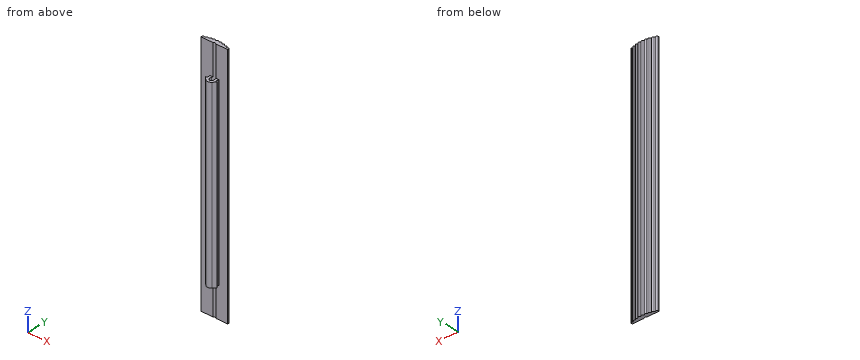
from build123d import *

# Parameters (mm, degrees)
BOSS_EXTRUDE2_DEPTH = 203.2
CUT_EXTRUDE1_REACH  = 357.917
SKETCH2_W           = 22.225
SKETCH2_H           = 25.4


with BuildPart() as part:
    # Sketch1 → Boss-Extrude2 (new body)
    with BuildSketch(Plane.XY.offset(152.4)):
        with BuildLine():
            Line((-11.1125, 7.155754294), (-11.1125, 6.2992))
            Line((-11.1125, 6.2992), (-4.0132, 6.2992))
            ThreePointArc((-4.0132, 6.2992), (-3.653989755, 6.150410245), (-3.5052, 5.7912))
            Line((-3.5052, 5.7912), (-3.5052, 3.980754294))
            ThreePointArc((-3.5052, 3.980754294), (-3.653989755, 3.621544049), (-4.0132, 3.472754294))
            Line((-4.0132, 3.472754294), (-4.7625, 3.472754294))
            Line((-4.7625, 3.472754294), (-2.563540889, 1.114659348))
            ThreePointArc((-2.563540889, 1.114659348), (1.91e-07, 0), (2.563541217, 1.114659472))
            Line((2.563541217, 1.114659472), (4.7625, 3.472754294))
            Line((4.7625, 3.472754294), (4.0132, 3.472754294))
            ThreePointArc((4.0132, 3.472754294), (3.653989755, 3.621544049), (3.5052, 3.980754294))
            Line((3.5052, 3.980754294), (3.5052, 5.7912))
            ThreePointArc((3.5052, 5.7912), (3.653989755, 6.150410245), (4.0132, 6.2992))
            Line((4.0132, 6.2992), (11.1125, 6.2992))
            Line((11.1125, 6.2992), (11.1125, 7.155754292))
            ThreePointArc((11.1125, 7.155754292), (10.663537153, 7.928210313), (9.770119113, 7.920454737))
            ThreePointArc((9.770119113, 7.920454737), (9.148763616, 7.659085907), (8.642363834, 8.104007899))
            ThreePointArc((8.642363834, 8.104007899), (8.019118897, 8.901877), (7.05308944, 8.59886472))
            ThreePointArc((7.05308944, 8.59886472), (6.504535766, 8.494192995), (6.085440415, 8.863281588))
            ThreePointArc((6.085440415, 8.863281588), (5.452899276, 9.555232733), (4.552056662, 9.295642159))
            ThreePointArc((4.552056662, 9.295642159), (3.931317659, 9.028192281), (3.421209266, 9.471628606))
            ThreePointArc((3.421209266, 9.471628606), (2.68084511, 9.976690828), (1.876956272, 9.580471612))
            ThreePointArc((1.876956272, 9.580471612), (1.327001325, 9.29621405), (0.796430567, 9.615192851))
            ThreePointArc((0.796430567, 9.615192851), (-2e-09, 10.1092), (-0.796430568, 9.615192848))
            ThreePointArc((-0.796430568, 9.615192848), (-1.327001326, 9.29621405), (-1.876956272, 9.580471612))
            ThreePointArc((-1.876956272, 9.580471612), (-2.680845114, 9.976690828), (-3.421209269, 9.471628598))
            ThreePointArc((-3.421209269, 9.471628598), (-3.931317662, 9.028192282), (-4.552056659, 9.295642158))
            ThreePointArc((-4.552056659, 9.295642158), (-5.45289928, 9.555232733), (-6.085440418, 8.863281574))
            ThreePointArc((-6.085440418, 8.863281574), (-6.504535766, 8.494192992), (-7.053089431, 8.59886471))
            ThreePointArc((-7.053089431, 8.59886471), (-8.019118881, 8.901877006), (-8.642363831, 8.104007918))
            ThreePointArc((-8.642363831, 8.104007918), (-9.148763609, 7.659085911), (-9.770119113, 7.920454739))
            ThreePointArc((-9.770119113, 7.920454739), (-10.663537153, 7.928210315), (-11.1125, 7.155754294))
        make_face()
        with BuildLine():
            Line((-1.5875, 3.472754294), (-1.5875, 5.276154294))
            ThreePointArc((-1.5875, 5.276154294), (0, 6.863654294), (1.5875, 5.276154294))
            Line((1.5875, 5.276154294), (1.5875, 3.472754294))
            ThreePointArc((1.5875, 3.472754294), (0, 1.885254294), (-1.5875, 3.472754294))
        make_face(mode=Mode.SUBTRACT)
    extrude(amount=BOSS_EXTRUDE2_DEPTH)

    # Cut-Extrude1: up to this face of the body (flat: up to its plane)
    cut_extrude1_end = Plane(part.part.faces().sort_by_distance((7.56285, 6.2992, 254))[0])
    # Sketch2 → Cut-Extrude1 (cut, up to the picked face)
    with BuildSketch(Plane(origin=(0, 0, 0), x_dir=(1, 0, 0), z_dir=(0, 1, 0)), mode=Mode.PRIVATE) as cut_extrude1_sk1:
        with Locations((0, -165.1)):
            Rectangle(SKETCH2_W, SKETCH2_H)
    cut_extrude1_tool1 = split(extrude(cut_extrude1_sk1.sketch, amount=CUT_EXTRUDE1_REACH, mode=Mode.PRIVATE), bisect_by=cut_extrude1_end, keep=Keep.BOTH, mode=Mode.PRIVATE)
    # Sketch2 → Cut-Extrude1 (cut, up to the picked face)
    with BuildSketch(Plane(origin=(0, 0, 0), x_dir=(1, 0, 0), z_dir=(0, 1, 0)), mode=Mode.PRIVATE) as cut_extrude1_sk2:
        with Locations((0, -342.9)):
            Rectangle(SKETCH2_W, SKETCH2_H)
    cut_extrude1_tool2 = split(extrude(cut_extrude1_sk2.sketch, amount=CUT_EXTRUDE1_REACH, mode=Mode.PRIVATE), bisect_by=cut_extrude1_end, keep=Keep.BOTH, mode=Mode.PRIVATE)
    add(cut_extrude1_tool1.solids().sort_by(Axis((0, 0, 165.1), (0, 1, 0)))[0], mode=Mode.SUBTRACT)
    add(cut_extrude1_tool2.solids().sort_by(Axis((0, 0, 342.9), (0, 1, 0)))[0], mode=Mode.SUBTRACT)


solid = part.part
Check sheet for the modelled part. Datum: model origin and axes. Units: mm. Give positions to 0.01 mm unless a question says otherwise; leave off trailing zeros. Write each loop counter-clockwise with the first axis right and the second up, starting at its lowest first coordinate (ties: lowest second). Pieces come first, ordered by that corner, then holes. Notation, with made-up numbers: M 33.5,20 L 92.5,20 A24 cw 92.5,44 Z; hole C -21,67.25 d7. An arc over 180 degrees is marked long. Use one line per item in the form item = value.
(1) Depth check by flat-ended pin: P1, Ø3, axis at x = -7, z = 221, coming from the +Y side; P2, Ø11, axis at x = 6, z = 292, coming from the -Y side; P3, Ø0.5, axis at y = 5, z = 227, coming from the -X side. Enter the tip coordinate at first touch or a pass-through.
Answer block:
P1 = 9.54
P2 = 0.04
P3 = -3.51
(2) Material ranges on line 1 along X through (y, z) = (5.5, 216); line 2 along X through (y, z) = (7.75, 330); line 3 along X through (y, z) = (8.75, 205.5), recorded low to high.
Answer block:
line_1 = -3.51 to -1.57, 1.57 to 3.51
line_2 = -10.88 to -9.59, -8.91 to 8.91, 9.59 to 10.88
line_3 = -8.31 to -7.2, -6.15 to 6.15, 7.2 to 8.31
(3) Section check A-A on z = 333. Record the boundary of the cut face in (x, y) (1 decimal), plus the area to 3 significant figures.
Answer block:
outline = M -11.1,6.3 L -1.2,6.3 A1.6 cw 1.2,6.3 L 11.1,6.3 L 11.1,7.2 A0.9 ccw 9.8,7.9 A0.6 cw 8.6,8.1 A0.9 ccw 7.1,8.6 A0.6 cw 6.1,8.9 A0.9 ccw 4.6,9.3 A0.6 cw 3.4,9.5 A0.9 ccw 1.9,9.6 A0.6 cw 0.8,9.6 A0.9 ccw -0.8,9.6 A0.6 cw -1.9,9.6 A0.9 ccw -3.4,9.5 A0.6 cw -4.6,9.3 A0.9 ccw -6.1,8.9 A0.6 cw -7.1,8.6 A0.9 ccw -8.6,8.1 A0.6 cw -9.8,7.9 A0.9 ccw -11.1,7.2 Z
area = 58.4 mm2
